```python
from build123d import *

# Parameters (mm, degrees)
BOSS_EXTRU_1_DEPTH      = 6
ESQUISSE2_W             = 8
ESQUISSE2_H             = 10
ENL_V_MAT_EXTRU_1_DEPTH = 2
ENL_V_MAT_EXTRU_2_DEPTH = 1
ENL_V_MAT_EXTRU_3_DEPTH = 1
BOSS_EXTRU_2_DEPTH      = 5
ENL_V_MAT_EXTRU_4_DEPTH = 6


with BuildPart() as part:
    # Esquisse1 → Boss.-Extru.1 (new body)
    with BuildSketch(Plane(origin=(0, 0, 0), x_dir=(1, 0, 0), z_dir=(0, 1, 0))):
        Polygon((-37.62183883, 41.220449501), (-54.508875838, -11.971243414), (-16.887037008, -53.191692914), (37.62183883, -41.220449501), (54.508875838, 11.971243414), (16.887037008, 53.191692914), align=None)
    extrude(amount=BOSS_EXTRU_1_DEPTH)

    # Esquisse2 → Enlèv. mat.-Extru.1 (cut)
    with BuildSketch(Plane(origin=(0, 6, 0), x_dir=(1, 0, 0), z_dir=(0, 1, 0))):
        Rectangle(ESQUISSE2_W, ESQUISSE2_H)
    extrude(amount=-ENL_V_MAT_EXTRU_1_DEPTH, mode=Mode.SUBTRACT)

    # Esquisse5 → Enlèv. mat.-Extru.2 (cut)
    with BuildSketch(Plane(origin=(0, 6, 0), x_dir=(1, 0, 0), z_dir=(0, 1, 0))):
        with BuildLine():
            Line((-2.5, 16.5), (-3.5, 0))
            Line((-3.5, 0), (-2.5, -16.5))
            ThreePointArc((-2.5, -16.5), (0, -19), (2.5, -16.5))
            Line((2.5, -16.5), (3.5, 0))
            Line((3.5, 0), (2.5, 16.5))
            ThreePointArc((2.5, 16.5), (0, 19), (-2.5, 16.5))
        make_face()
    extrude(amount=-ENL_V_MAT_EXTRU_2_DEPTH, mode=Mode.SUBTRACT)

    # Esquisse6 → Enlèv. mat.-Extru.3 (cut)
    with BuildSketch(Plane(origin=(0, 6, 0), x_dir=(1, 0, 0), z_dir=(0, 1, 0))):
        with BuildLine():
            Line((-5.05, 2), (5.05, 2))
            ThreePointArc((5.05, 2), (7.05, 0), (5.05, -2))
            Line((5.05, -2), (-5.05, -2))
            ThreePointArc((-5.05, -2), (-7.05, 0), (-5.05, 2))
        make_face()
    extrude(amount=-ENL_V_MAT_EXTRU_3_DEPTH, mode=Mode.SUBTRACT)

    # Esquisse7 → Boss.-Extru.2 (add)
    with BuildSketch(Plane(origin=(0, 6, 0), x_dir=(1, 0, 0), z_dir=(0, 1, 0))):
        with BuildLine():
            Line((-2.5, 16.5), (-2.696377272, 13.259775018))
            ThreePointArc((-2.696377272, 13.259775018), (-13.53115235, 0), (-2.696377272, -13.259775018))
            Line((-2.696377272, -13.259775018), (-2.5, -16.5))
            ThreePointArc((-2.5, -16.5), (-16.688319268, 0), (-2.5, 16.5))
        make_face()
        with BuildLine():
            Line((2.5, 16.5), (2.696377272, 13.259775018))
            ThreePointArc((2.696377272, 13.259775018), (13.53115235, 0), (2.696377272, -13.259775018))
            Line((2.696377272, -13.259775018), (2.5, -16.5))
            ThreePointArc((2.5, -16.5), (16.688319268, 0), (2.5, 16.5))
        make_face()
    extrude(amount=BOSS_EXTRU_2_DEPTH)

    # Esquisse8 → Enlèv. mat.-Extru.4 (cut)
    with BuildSketch(Plane(origin=(0, 6, 0), x_dir=(1, 0, 0), z_dir=(0, 1, 0))):
        with BuildLine():
            ThreePointArc((-46.080402753, -3.15609697), (-47.261935037, -10.79446929), (-42.696259662, -17.031083645))
            ThreePointArc((-42.696259662, -17.031083645), (-40.497960079, -16.494913015), (-41.034130709, -14.296613432))
            ThreePointArc((-41.034130709, -14.296613432), (-44.153069953, -10.036209514), (-43.345932541, -4.818225923))
            ThreePointArc((-43.345932541, -4.818225923), (-43.882103171, -2.61992634), (-46.080402753, -3.15609697))
        make_face()
        with BuildLine():
            ThreePointArc((-25.773461529, 38.328750916), (-32.979252144, 35.532801729), (-36.097480922, 28.460503691))
            ThreePointArc((-36.097480922, 28.460503691), (-34.533993744, 26.824805722), (-32.898295775, 28.3882929))
            ThreePointArc((-32.898295775, 28.3882929), (-30.768147373, 33.219575477), (-25.845672321, 35.12956577))
            ThreePointArc((-25.845672321, 35.12956577), (-24.209974352, 36.693052947), (-25.773461529, 38.328750916))
        make_face()
        with BuildLine():
            ThreePointArc((20.306941224, 41.484847886), (14.282682893, 46.327271019), (6.59877874, 45.491587336))
            ThreePointArc((6.59877874, 45.491587336), (5.963966335, 43.319718738), (8.135834934, 42.684906333))
            ThreePointArc((8.135834934, 42.684906333), (13.38492258, 43.255784991), (17.50026022, 39.947791692))
            ThreePointArc((17.50026022, 39.947791692), (19.672128819, 39.312979287), (20.306941224, 41.484847886))
        make_face()
        with BuildLine():
            ThreePointArc((46.080402753, 3.15609697), (47.261935037, 10.79446929), (42.696259662, 17.031083645))
            ThreePointArc((42.696259662, 17.031083645), (40.497960079, 16.494913015), (41.034130709, 14.296613432))
            ThreePointArc((41.034130709, 14.296613432), (44.153069953, 10.036209514), (43.345932541, 4.818225923))
            ThreePointArc((43.345932541, 4.818225923), (43.882103171, 2.61992634), (46.080402753, 3.15609697))
        make_face()
        with BuildLine():
            ThreePointArc((25.773461529, -38.328750916), (32.979252144, -35.532801729), (36.097480922, -28.460503691))
            ThreePointArc((36.097480922, -28.460503691), (34.533993744, -26.824805722), (32.898295775, -28.3882929))
            ThreePointArc((32.898295775, -28.3882929), (30.768147373, -33.219575477), (25.845672321, -35.12956577))
            ThreePointArc((25.845672321, -35.12956577), (24.209974352, -36.693052947), (25.773461529, -38.328750916))
        make_face()
        with BuildLine():
            ThreePointArc((-20.306941224, -41.484847886), (-14.282682893, -46.327271019), (-6.59877874, -45.491587336))
            ThreePointArc((-6.59877874, -45.491587336), (-5.963966335, -43.319718738), (-8.135834934, -42.684906333))
            ThreePointArc((-8.135834934, -42.684906333), (-13.38492258, -43.255784991), (-17.50026022, -39.947791692))
            ThreePointArc((-17.50026022, -39.947791692), (-19.672128819, -39.312979287), (-20.306941224, -41.484847886))
        make_face()
    extrude(amount=-ENL_V_MAT_EXTRU_4_DEPTH, mode=Mode.SUBTRACT)


solid = part.part
```
The model under review builds one solid part; all positions refer to its coordinate system, in mm. A direction names the side the tool comes from. Give positions to 0.01 mm unless a question says otherwise; leave off trailing zeros. Write each loop counter-clockwise with the first axis right and the second up, starting at its lowest first coordinate (ties: lowest second). Pieces come first, ordered by that corner, then holes. Notation, with made-up numbers: M 80,-37 L 98,-37 A10 ccw 98,-29 Z; hole C -9,-16 d8. An arc over 180 degrees is marked long. Answer in a Markdown table with one row per item.
Item 1: Add section A-A on y = 7.5. Give the boundary of the cut face in (x, z).
Check sheet entries:
| item | result |
|---|---|
| outline | M -2.7,-13.26 A13.53 cw -2.7,13.26 L -2.5,16.5 A16.69 ccw -2.5,-16.5 Z; M 2.5,-16.5 A16.69 ccw 2.5,16.5 L 2.7,13.26 A13.53 cw 2.7,-13.26 Z |
Item 2: For line 1 along X through (y, z) = (5.5, 13); line 2 along Y through (x, z) = (-32, 0.5); line 3 along Z through (x, y) = (26, 3.5), list the stretches that pass through material, from the lowest coordinate up.
Check sheet entries:
| item | result |
|---|---|
| line 1 | -53.57 to -46.44, -42.59 to -2.71, 2.71 to 46.58 |
| line 2 | 0 to 6 |
| line 3 | -43.21 to 35.13, 38.33 to 43.77 |
Item 3: Add section D-D on z = 0. Give the boundary of the cut face in (x, y), plus the area to 3 significant figures.
Check sheet entries:
| item | result |
|---|---|
| outline | M -50.71,0 L 50.71,0 L 50.71,6 L 16.69,6 L 16.69,11 L 13.53,11 L 13.53,6 L 7.05,6 L 7.05,5 L 4,5 L 4,4 L -4,4 L -4,5 L -7.05,5 L -7.05,6 L -13.53,6 L -13.53,11 L -16.69,11 L -16.69,6 L -50.71,6 Z |
| area | 618 mm2 |
Item 4: Tool access review of faces 1 (the face through (11, 6, -13)), 2 (the face through (34.569, 3.042, 26.826)): name each direction out of +Z, -Z, +X, -X, +Y, -Y from which nothing blocks a thin tool from reaching the whole face with its end or side.
Check sheet entries:
| item | result |
|---|---|
| face 1 | +Y |
| face 2 | +Y, -Y |
Item 5: Add section B-B on x = -28. Give the boundary of the cut face in (y, z), plus the area to 3 significant figures.
Check sheet entries:
| item | result |
|---|---|
| outline | M 0,-43.33 L 6,-43.33 L 6,-38.13 L 0,-38.13 Z; M 0,-34.84 L 6,-34.84 L 6,41.02 L 0,41.02 Z |
| area | 486 mm2 |
Item 6: Draft analysis for pull direction X (two halves, no side actions). For faces 3 (the face through (-45.947, 2.958, -14.997)), 4 (the face through (-1, 0, -1)), 5 (the face through (45.947, 2.958, 14.997)), 6 (the face through (13.312, 3.042, -43.277)), state which applies: +X half, -X half, draft (parallel to the pull), parting line (faces both ways), or undercut.
Check sheet entries:
| item | result |
|---|---|
| face 3 | -X half |
| face 4 | draft |
| face 5 | +X half |
| face 6 | undercut |
Item 7: For P1, Ø0.5, axis at x = 4.5, y = 5.5, coming from the +Z side; P2, Ø3, axis at x = 29, y = 3.5, coming from the +Z side; P3, Ø2, axis at x = -1, y = 4.5, coming from the +Z side; P4, Ø2, axis at y = 8.5, z = -35.5, coming from the -X side, all flat-tipped, find the tip position at first contact; note any pin that passes through.
Check sheet entries:
| item | result |
|---|---|
| P1 | z = 48.55 |
| P2 | z = 43.44 |
| P3 | z = 49.92 |
| P4 | through |
Item 8: Add section C-C on y = 1.25. State how many separate pieces and enclosed holes the cut face has, plus the area to 3 significant figures.
Check sheet entries:
| item | result |
|---|---|
| separate pieces | 1 |
| enclosed holes | 6 |
| area | 7,790 mm2 |
